Could you check a few things on this model? Use its own coordinates, in mm. Face numbers are marked on the shaded views. A direction names the side the tool comes from. Round coordinates to 2 decimals unless told otherwise and drop trailing zeros. Write each loop counter-clockwise with the first axis right and the second up, starting at its lowest first coordinate (ties: lowest second). Pieces come first, ordered by that corner, then holes. Notation, with made-up numbers: (36.25, 13) -> (76.25, 13) arc R11 ccw to (76.25, 28) -> close; hole circle Ø5 at (67.5, 77). An arc over 180 degrees is marked (long way). Return JSON: item names as keys, results as strings.
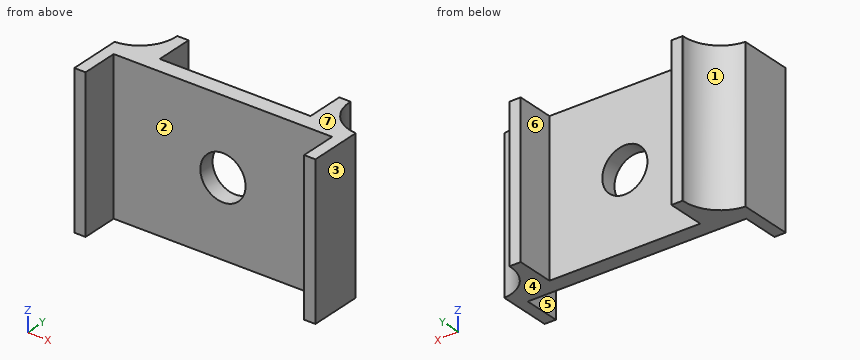
from build123d import *

# Parameters (mm, degrees)
F1_DEPTH    = 20
F2_T1_DEPTH = 20
F3_R        = 3
F4_DEPTH    = 25


# Not quite as in the source:
# - a fillet or chamfer that OpenCascade refuses, or shapes differently, is made with other operations: its cross-section is extruded or revolved along the edge and cut away or added


with BuildPart() as f1:
    # F0 (on Top) → F1 (new body)
    with BuildSketch(Plane.XY):
        Polygon((0, -7), (0, 0), (-4.5, 0), (-4.5, 5), (-6, 5), (-6, 0), (-26, 0), (-26, 5), (-27.5, 5), (-27.5, 0), (-32, 0), (-32, -7), (-30.5, -7), (-30.5, -2.1179924456), (-1.5, -2.1179924456), (-1.5, -7), align=None)
    extrude(amount=F1_DEPTH)

    # F2: fillet of radius 4.8260129112 on 2 edges, made by hand

    # F2_s2 → F2_t1 (join)
    with BuildSketch(Plane.XY):
        with BuildLine():
            ThreePointArc((-27.5, 4.814988702), (-28.8001269844, 1.5197604777), (-32, 0))
            Line((-32, 0), (-27.5, 0))
            Line((-27.5, 0), (-27.5, 4.814988702))
        make_face()
        with BuildLine():
            ThreePointArc((0, 0), (-3.1998730156, 1.5197604777), (-4.5, 4.814988702))
            Line((-4.5, 4.814988702), (-4.5, 0))
            Line((-4.5, 0), (0, 0))
        make_face()
    extrude(amount=F2_T1_DEPTH)

    # F3 (on face) → F4 (cut)
    with BuildSketch(Plane.XZ.offset(2.1179924456)):
        with Locations((-16, 10)):
            Circle(F3_R)
    extrude(amount=-F4_DEPTH, mode=Mode.SUBTRACT)


solid = f1.part
1) I want a section at D-D, the plane z = 17. Please give me the cut outline in (x, y).
Return value:
{"outline": "(-32, -7) -> (-30.5, -7) -> (-30.5, -2.12) -> (-1.5, -2.12) -> (-1.5, -7) -> (0, -7) -> (0, 0) arc R4.83 cw to (-4.5, 4.81) -> (-4.5, 5) -> (-6, 5) -> (-6, 0) -> (-26, 0) -> (-26, 5) -> (-27.5, 5) -> (-27.5, 4.81) arc R4.83 cw to (-32, 0) -> close"}
2) Thinking about a two-plate mould opening in X: for the marked faces 1, 2, 3 and 4, which applies, pulls with the +X half, pulls with the -X half, needs draft (parallel to the pull), parting line crosses it, or undercut?
Return value:
{"face 1": "pulls with the -X half", "face 2": "undercut", "face 3": "pulls with the +X half", "face 4": "needs draft"}
3) For the marked faces 5, 6 and 7, which set-ups out of +Z, -Z, +X, -X, +Y, -Y let a thin tool reach every point of the face, with its end or its side?
Return value:
{"face 5": "+Z, -Z, -Y", "face 6": "+Z, -Z, +Y", "face 7": "+Z, +X, -X, +Y, -Y"}
4) Will these pins go through, and if not, where does the flat tip stop? pin 1 Ø6 at (x, z) = (-11.5, 7) entering from -Y; pin 2 Ø7 at (x, z) = (-16, 10) entering from +Y.
Return value:
{"pin 1": "y = -2.12", "pin 2": "y = 0"}
5) I want a section at A-A, the plane x = -16. Please give me the cut outline in (y, z).
Return value:
{"outline": "(-2.12, 0) -> (0, 0) -> (0, 7) -> (-2.12, 7) -> close; (-2.12, 13) -> (0, 13) -> (0, 20) -> (-2.12, 20) -> close"}
6) I want a section at C-C, the plane z = 10. Please give me the cut outline in (x, y), and give its area (3 significant figures).
Return value:
{"outline": "(-32, -7) -> (-30.5, -7) -> (-30.5, -2.12) -> (-19, -2.12) -> (-19, 0) -> (-26, 0) -> (-26, 5) -> (-27.5, 5) -> (-27.5, 4.81) arc R4.83 cw to (-32, 0) -> close; (-13, -2.12) -> (-1.5, -2.12) -> (-1.5, -7) -> (0, -7) -> (0, 0) arc R4.83 cw to (-4.5, 4.81) -> (-4.5, 5) -> (-6, 5) -> (-6, 0) -> (-13, 0) -> close", "area": "94.6 mm²"}
7) I want a section at B-B, the plane y = -6. Please give me the cut outline in (x, z), and give its area (3 significant figures).
Return value:
{"outline": "(-32, 0) -> (-30.5, 0) -> (-30.5, 20) -> (-32, 20) -> close; (-1.5, 0) -> (0, 0) -> (0, 20) -> (-1.5, 20) -> close", "area": "60.0 mm²"}
8) If I drill on probe 1 along Z at (x, y) = (-16, -1.5); probe 2 along X at (y, z) = (-3.5, 2.5); probe 3 along Y at (x, z) = (-23.5, 4.25), over which ranges is the centre line in solid material (lowest first)? Write a range as [from, to].
Return value:
{"probe 1": "[0, 7], [13, 20]", "probe 2": "[-32, -30.5], [-1.5, 0]", "probe 3": "[-2.12, 0]"}
